```python
from build123d import *

# Parameters (mm, degrees)
SKETCH1_W           = 60
SKETCH1_H           = 40
BOSS_EXTRUDE1_DEPTH = 0.5
SKETCH2_R           = 1.5
CUT_EXTRUDE1_DEPTH  = 1
SKETCH3_W           = 46
SKETCH3_H           = 8
BOSS_EXTRUDE2_DEPTH = 6
CUT_EXTRUDE2_DEPTH  = 59.139917441


with BuildPart() as part:
    # Sketch1 → Boss-Extrude1 (new, symmetric)
    with BuildSketch(Plane(origin=(0, 0, 0), x_dir=(1, 0, 0), z_dir=(0, 1, 0))):
        Rectangle(SKETCH1_W, SKETCH1_H)
    extrude(amount=BOSS_EXTRUDE1_DEPTH, both=True)

    # Sketch2 → Cut-Extrude1 (cut)
    with BuildSketch(Plane(origin=(0, 0.5, 0), x_dir=(1, 0, 0), z_dir=(0, 1, 0))):
        with Locations(Location((-28, 18, 0), (0, 0, 270))):
            Circle(SKETCH2_R)
        with Locations(Location((28, 18, 0), (0, 0, 90))):
            Circle(SKETCH2_R)
        with Locations(Location((28, -18, 0), (0, 0, 270))):
            Circle(SKETCH2_R)
        with Locations(Location((-28, -18, 0), (0, 0, 90))):
            Circle(SKETCH2_R)
    extrude(amount=-CUT_EXTRUDE1_DEPTH, mode=Mode.SUBTRACT)

    # Sketch3 → Boss-Extrude2 (add)
    with BuildSketch(Plane(origin=(0, 0.5, 0), x_dir=(1, 0, 0), z_dir=(0, 1, 0))):
        with Locations((0, 19)):
            Rectangle(SKETCH3_W, SKETCH3_H)
    extrude(amount=BOSS_EXTRUDE2_DEPTH)

    # Sketch4 → Cut-Extrude2 (cut, through all)
    with BuildSketch(Plane(origin=(23, 0, 0), x_dir=(0, 0, -1), z_dir=(1, 0, 0))):
        Polygon((23, 5.2), (23, 6.5), (20.2, 6.5), align=None)
        Polygon((20.2, 0.5), (23, 1.8), (23, 0.5), align=None)
    extrude(amount=-CUT_EXTRUDE2_DEPTH, mode=Mode.SUBTRACT)


solid = part.part
```
Can you work these out from the model? Positions are in its coordinate system, mm. A direction names the side the tool comes from. Round coordinates to 2 decimals unless told otherwise and drop trailing zeros. Loops run counter-clockwise (first coordinate to the right, second up) from the corner with the lowest first, then second, coordinate; pieces in that order, holes last.
Item 1: Which directions (+Z, -Z, +X, -X, +Y, -Y) give clear straight access to the entire face, cutting with the end or side of a thin tool? Please do faces 4 (the cylindrical face through (-26.99, 0.01, -19.11)), 5 (the flat face through (0, 3, -15)), 6 (the flat face through (23, 3, -19)).
Item 2: Will these pins go through, and if not, where does the flat tip stop? pin 1 Ø1.5 at (x, y) = (18.5, 3.5) entering from +Z; pin 2 Ø20 at (x, z) = (7, -0.5) entering from +Y; pin 3 Ø1.8 at (y, z) = (3.5, -18) entering from -X.
Item 3: Suppose I cut it at D-D, the plane y = 3. Write out the boundary of the cut face in (x, z), then the cut area to 3 significant figures.
Item 4: Please list where these lines run through material, in increasing order: L1, parallel to X at y = 0.15, z = 18; L2, parallel to Y at x = -17, z = -8; L3, parallel to Z at x = -20, y = 4.
Item 5: Suppose I cut it at A-A, the plane x = -28. Write out the boundary of the cut face in (y, z), then the cut area to 3 significant figures.
Item 6: Suppose I cut it at C-C, the plane z = -18. Write out the boundary of the cut face in (x, y).
Item 7: If we mould it in two halves opening along X, with no side actions, what happens to faces 1 (the cylindrical face through (26.99, 0.01, -16.89)), 2 (the flat face through (-23, 3, -19)), 3 (the flat face through (0, -0.5, 0))? For each: +X half, -X half, draft (parallel to the pull), parting line (faces both ways), or undercut.
Item 8: Suppose I cut it at B-B, the plane z = 18. Write out the boundary of the cut face in (x, y), then the cut area to 3 significant figures.
Reported:
1. face 4: +Y, -Y
1. face 5: +Z, +X, -X, +Y
1. face 6: +Z, -Z, +X, +Y
2. pin 1: stops at z = -15
2. pin 2: stops at y = 0.5
2. pin 3: stops at x = -23
3. outline: (-23, -23) - (23, -23) - (23, -15) - (-23, -15) - close
3. area: 368 mm2
4. L1: x = -30 to -29.5, -26.5 to 26.5, 29.5 to 30
4. L2: y = -0.5 to 0.5
4. L3: z = -23 to -15
5. outline: (-0.5, -20) - (0.5, -20) - (0.5, -19.5) - (-0.5, -19.5) - close; (-0.5, -16.5) - (0.5, -16.5) - (0.5, 16.5) - (-0.5, 16.5) - close; (-0.5, 19.5) - (0.5, 19.5) - (0.5, 20) - (-0.5, 20) - close
5. area: 34.0 mm2
6. outline: (-30, -0.5) - (-29.5, -0.5) - (-29.5, 0.5) - (-30, 0.5) - close; (-26.5, -0.5) - (26.5, -0.5) - (26.5, 0.5) - (23, 0.5) - (23, 6.5) - (-23, 6.5) - (-23, 0.5) - (-26.5, 0.5) - close; (29.5, -0.5) - (30, -0.5) - (30, 0.5) - (29.5, 0.5) - close
7. face 1: undercut
7. face 2: -X half
7. face 3: draft
8. outline: (-30, -0.5) - (-29.5, -0.5) - (-29.5, 0.5) - (-30, 0.5) - close; (-26.5, -0.5) - (26.5, -0.5) - (26.5, 0.5) - (-26.5, 0.5) - close; (29.5, -0.5) - (30, -0.5) - (30, 0.5) - (29.5, 0.5) - close
8. area: 54.0 mm2
